from build123d import *

# Parameters (mm, degrees)
F3_W     = 21.7424
F3_H     = 5.08
F4_DEPTH = 5.073509


with BuildPart() as f1:
    # F0 (on Front) → F1 (revolve)
    with BuildSketch(Plane.XZ):
        with BuildLine():
            Line((0, 30.980509), (0, 0))
            Line((0, 0), (6.35, 0))
            Line((6.35, 0), (6.35, 24.625533))
            Line((6.35, 24.625533), (12.509782, 24.625533))
            ThreePointArc((12.509782, 24.625533), (7.015703, 29.300681), (0, 30.980509))
        make_face()
        Polygon((6.35, 0), (0, 0), (0, -3.81), (4.250277, -3.81), align=None)
    revolve(axis=Axis((0, 0, 15.490254), (0, 0, 1)))

    # F3 (on offset) → F4 (cut, through all)
    with BuildSketch(Plane.XY.offset(25.908)):
        Rectangle(F3_W, F3_H)
    extrude(amount=F4_DEPTH, mode=Mode.SUBTRACT)


solid = f1.part
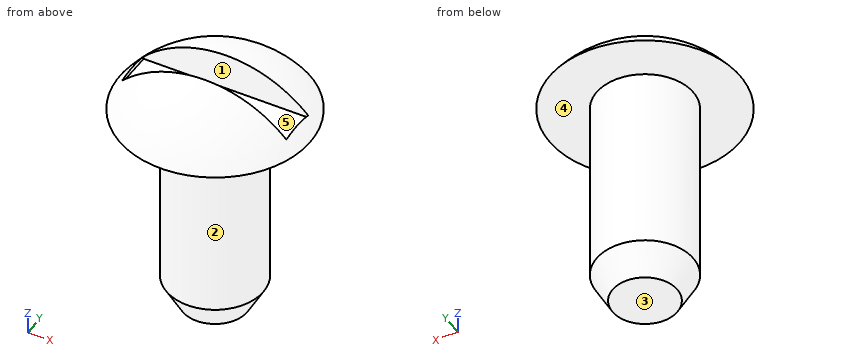
Model file for the job. Use its own axes, mm. Face numbers are marked on the shaded views. A direction names the side the tool comes from. Give positions to 0.01 mm unless a question says otherwise; leave off trailing zeros. Loops run counter-clockwise (first coordinate to the right, second up) from the corner with the lowest first, then second, coordinate; pieces in that order, holes last. Notation, with made-up numbers: (86.25, 28.25) -> (93.25, 28.25) arc R31 cw to (93.25, 54.25) -> close; hole circle Ø9 at (56, 55.5). An arc over 180 degrees is marked (long way). Use a Markdown table: item, result. Add a question column.
(1) Slice it at B-B on z = -1. List the corners of the cut face in (x, y), and give its area (3 significant figures).
(2) Mould opens along Y. For the marked faces 1, 2 and 3 say: +Y half, -Y half, draft (parallel to the pull), parting line (faces both ways), or undercut.
(3) Slice it at A-A on z = 18.5. List the corners of the cut face in (x, y), and give its area (3 significant figures).
(4) Drop flat-ended pins along their axis: pin 1 Ø1.5 at (x, z) = (-5, 26.5) entering from -Y; pin 2 Ø8 at (x, y) = (-1.5, 3.5) entering from +Z; pin 3 Ø2.5 at (x, z) = (-1.5, 27.5) entering from -Y; pin 4 Ø2.5 at (x, z) = (-1.5, 29) entering from +Y. Give the stop position or say it passes through.
(5) Tool access for the marked faces 4 and 5: list every direction of +Z, -Z, +X, -X, +Y, -Y with a clear straight run to the whole face (end or side of a thin tool).
(6) Wall check: line 1 along Z through (x, y) = (0, -0.75); line 2 along Y through (x, z) = (4.5, 28.5); line 3 along Z through (x, y) = (-10.5, 1.5). Give the ranges that are in metal, low to high.
Filled sheet:
| question | item | result |
|---|---|---|
| 1 | outline | circle Ø11.6 at (0, 0) |
| 1 | area | 106 mm2 |
| 2 | face 1 | undercut |
| 2 | face 2 | parting line |
| 2 | face 3 | draft |
| 3 | outline | circle Ø12.7 at (0, 0) |
| 3 | area | 127 mm2 |
| 4 | pin 1 | y = -10.55 |
| 4 | pin 2 | z = 30.77 |
| 4 | pin 3 | y = -11.05 |
| 4 | pin 4 | y = 9.36 |
| 5 | face 4 | -Z |
| 5 | face 5 | +Z |
| 6 | line 1 | -3.81 to 25.91 |
| 6 | line 2 | -7.1 to -2.54, 2.54 to 7.1 |
| 6 | line 3 | 24.63 to 25.91 |
